from build123d import *

# Parameters (mm, degrees)
SKIZZE1_W                        = 150
SKIZZE1_H                        = 150
AUFSATZ_LINEAR_AUSTRAGEN1_DEPTH  = 2
AUFSATZ_LINEAR_AUSTRAGEN2_DEPTH  = 80
SCHNITT_LINEAR_AUSTRAGEN1_DEPTH  = 10
SKIZZE5_W                        = 17
SKIZZE5_H                        = 13
SCHNITT_LINEAR_AUSTRAGEN3_DEPTH  = 10
SKIZZE6_W                        = 17
SKIZZE6_H                        = 19
SCHNITT_LINEAR_AUSTRAGEN4_DEPTH  = 2
SKIZZE7_W                        = 17
SKIZZE7_H                        = 3
SCHNITT_LINEAR_AUSTRAGEN5_DEPTH  = 10
SKIZZE9_W                        = 18
SKIZZE9_H                        = 21
AUFSATZ_LINEAR_AUSTRAGEN3_DEPTH  = 63
SKIZZE10_W                       = 15
SKIZZE10_H                       = 10
SCHNITT_LINEAR_AUSTRAGEN6_DEPTH  = 63
SCHNITT_LINEAR_AUSTRAGEN7_DEPTH  = 2
SKIZZE17_R                       = 1
SCHNITT_LINEAR_AUSTRAGEN10_DEPTH = 1
SKIZZE18_W                       = 7
SKIZZE18_H                       = 7
SCHNITT_LINEAR_AUSTRAGEN11_DEPTH = 4.5
SKIZZE19_R                       = 0.9
SCHNITT_LINEAR_AUSTRAGEN12_DEPTH = 15
SKIZZE20_W                       = 25
SKIZZE20_H                       = 37
SCHNITT_LINEAR_AUSTRAGEN13_DEPTH = 4
SKIZZE21_W                       = 7
SKIZZE21_H                       = 37
SCHNITT_LINEAR_AUSTRAGEN14_DEPTH = 3
SCHNITT_LINEAR_AUSTRAGEN15_DEPTH = 6


with BuildPart() as part:
    # Skizze1 → Aufsatz-Linear austragen1 (new body)
    with BuildSketch(Plane(origin=(0, 0, 0), x_dir=(1, 0, 0), z_dir=(0, 1, 0))):
        with Locations((-0.733702775, 32.058376742)):
            Rectangle(SKIZZE1_W, SKIZZE1_H)
    extrude(amount=-AUFSATZ_LINEAR_AUSTRAGEN1_DEPTH)

    # Skizze1_3 → Aufsatz-Linear austragen2 (add)
    with BuildSketch(Plane(origin=(0, 0, 0), x_dir=(1, 0, 0), z_dir=(0, 1, 0))):
        Polygon((-75.733702775, 107.058376742), (-75.733702775, 48.496785112), (-70.733702775, 48.496785112), (-70.733702775, 105.058376742), (69.266297225, 105.058376742), (69.266297225, 56.802887669), (74.266297225, 56.802887669), (74.266297225, 107.058376742), align=None)
        Polygon((-15.65559864, -40.941623258), (-15.65559864, -42.941623258), (74.266297225, -42.941623258), (74.266297225, 56.802887669), (69.266297225, 56.802887669), (69.266297225, -40.941623258), align=None)
        Polygon((-70.733702775, 48.496785112), (-75.733702775, 48.496785112), (-75.733702775, -42.941623258), (-15.65559864, -42.941623258), (-15.65559864, -40.941623258), (-70.733702775, -40.941623258), align=None)
    extrude(amount=AUFSATZ_LINEAR_AUSTRAGEN2_DEPTH)

    # Skizze2 → Schnitt-Linear austragen1 (cut)
    with BuildSketch(Plane.ZY.offset(75.733702775)):
        Polygon((-75.558376742, 67.5), (-75.558376742, 62.78), (-32.058376742, 39), (11.441623258, 62.78), (11.441623258, 67.5), align=None)
        Polygon((-32.058376742, 39), (-75.558376742, 62.78), (-75.558376742, 15.22), align=None)
        Polygon((11.441623258, 15.22), (-32.058376742, 39), (-75.558376742, 15.22), (-75.558376742, 10.5), (11.441623258, 10.5), align=None)
        Polygon((11.441623258, 62.78), (-32.058376742, 39), (11.441623258, 15.22), align=None)
    extrude(amount=-SCHNITT_LINEAR_AUSTRAGEN1_DEPTH, mode=Mode.SUBTRACT)

    # Skizze5 → Schnitt-Linear austragen3 (cut)
    with BuildSketch(Plane(origin=(74.266297225, 0, 0), x_dir=(0, 0, -1), z_dir=(1, 0, 0))):
        with Locations((93.558376742, 68.5)):
            Rectangle(SKIZZE5_W, SKIZZE5_H)
    extrude(amount=-SCHNITT_LINEAR_AUSTRAGEN3_DEPTH, mode=Mode.SUBTRACT)

    # Skizze6 → Schnitt-Linear austragen4 (cut)
    with BuildSketch(Plane(origin=(74.266297225, 0, 0), x_dir=(0, 0, -1), z_dir=(1, 0, 0))):
        with Locations((-29.441623258, 65.5)):
            Rectangle(SKIZZE6_W, SKIZZE6_H)
    extrude(amount=-SCHNITT_LINEAR_AUSTRAGEN4_DEPTH, mode=Mode.SUBTRACT)

    # Skizze7 → Schnitt-Linear austragen5 (cut)
    with BuildSketch(Plane(origin=(72.266297225, 0, 0), x_dir=(0, 0, -1), z_dir=(1, 0, 0))):
        with Locations((-29.441623258, 73.5)):
            Rectangle(SKIZZE7_W, SKIZZE7_H)
    extrude(amount=-SCHNITT_LINEAR_AUSTRAGEN5_DEPTH, mode=Mode.SUBTRACT)

    # Skizze9 → Aufsatz-Linear austragen3 (add)
    with BuildSketch(Plane(origin=(0, 0, 0), x_dir=(1, 0, 0), z_dir=(0, 1, 0))):
        with Locations((60.266297225, 94.558376742)):
            Rectangle(SKIZZE9_W, SKIZZE9_H)
    extrude(amount=AUFSATZ_LINEAR_AUSTRAGEN3_DEPTH)

    # Skizze10 → Schnitt-Linear austragen6 (cut)
    with BuildSketch(Plane(origin=(0, 0, 40.941623258), x_dir=(-1, 0, 0), z_dir=(0, 0, -1))):
        with Locations((-61.766297225, 5)):
            Rectangle(SKIZZE10_W, SKIZZE10_H)
    extrude(amount=-SCHNITT_LINEAR_AUSTRAGEN6_DEPTH, mode=Mode.SUBTRACT)

    # Skizze11 → Schnitt-Linear austragen7 (cut)
    with BuildSketch(Plane(origin=(-70.733702775, 0, 0), x_dir=(0, 0, -1), z_dir=(1, 0, 0))):
        Polygon((75.558376742, 16.164383562), (32.058376742, 40), (-11.441623258, 16.164383562), (-11.441623258, 10.5), (75.558376742, 10.5), align=None)
        Polygon((75.558376742, 63.835616438), (32.058376742, 40), (75.558376742, 16.164383562), align=None)
        Polygon((-11.441623258, 67.5), (-11.441623258, 63.835616438), (32.058376742, 40), (75.558376742, 63.835616438), (75.558376742, 67.5), align=None)
        Polygon((32.058376742, 40), (-11.441623258, 63.835616438), (-11.441623258, 16.164383562), align=None)
        Polygon((-11.441623258, 63.835616438), (-18.441623258, 67.671232877), (-18.441623258, 12.328767123), (-11.441623258, 16.164383562), align=None)
        Polygon((-18.441623258, 72.5), (-18.441623258, 67.671232877), (-11.441623258, 63.835616438), (-11.441623258, 67.5), (75.558376742, 67.5), (75.558376742, 63.835616438), (82.558376742, 67.671232877), (82.558376742, 72.5), align=None)
        Polygon((75.558376742, 63.835616438), (75.558376742, 16.164383562), (82.558376742, 12.328767123), (82.558376742, 67.671232877), align=None)
        Polygon((-11.441623258, 16.164383562), (-18.441623258, 12.328767123), (-18.441623258, 7.5), (82.558376742, 7.5), (82.558376742, 12.328767123), (75.558376742, 16.164383562), (75.558376742, 10.5), (-11.441623258, 10.5), align=None)
    extrude(amount=-SCHNITT_LINEAR_AUSTRAGEN7_DEPTH, mode=Mode.SUBTRACT)

    # Skizze17 → Schnitt-Linear austragen10 (cut)
    with BuildSketch(Plane(origin=(-72.733702775, 0, 0), x_dir=(0, 0, -1), z_dir=(1, 0, 0))):
        with Locations((77.758376742, 67)):
            Circle(SKIZZE17_R)
        with Locations((77.758376742, 11)):
            Circle(SKIZZE17_R)
        with Locations((-13.641623258, 11)):
            Circle(SKIZZE17_R)
        with Locations((-13.641623258, 67)):
            Circle(SKIZZE17_R)
    extrude(amount=-SCHNITT_LINEAR_AUSTRAGEN10_DEPTH, mode=Mode.SUBTRACT)

    # Skizze18 → Schnitt-Linear austragen11 (cut)
    with BuildSketch(Plane.ZY.offset(75.733702775)):
        with Locations((27.191623258, 57.5)):
            Rectangle(SKIZZE18_W, SKIZZE18_H)
        Polygon((30.691623258, 31), (27.191623258, 31), (23.691623258, 31), (23.691623258, 24), (30.691623258, 24), align=None)
        with Locations((27.191623258, 37.5)):
            Rectangle(SKIZZE18_W, SKIZZE18_H)
        with Locations((27.191623258, 47.5)):
            Rectangle(SKIZZE18_W, SKIZZE18_H)
        with Locations((-91.518407477, 57.5)):
            Rectangle(SKIZZE18_W, SKIZZE18_H)
        with Locations((-91.518407477, 47.5)):
            Rectangle(SKIZZE18_W, SKIZZE18_H)
        with Locations((-91.518407477, 37.5)):
            Rectangle(SKIZZE18_W, SKIZZE18_H)
        with Locations((-91.518407477, 27.5)):
            Rectangle(SKIZZE18_W, SKIZZE18_H)
    extrude(amount=-SCHNITT_LINEAR_AUSTRAGEN11_DEPTH, mode=Mode.SUBTRACT)

    # Skizze19 → Schnitt-Linear austragen12 (cut)
    with BuildSketch(Plane(origin=(0, 80, 0), x_dir=(1, 0, 0), z_dir=(0, 1, 0))):
        with BuildLine():
            Line((72.666297225, 7.058376742), (71.766297225, 7.058376742))
            Line((71.766297225, 7.058376742), (71.766297225, 6.158376742))
            ThreePointArc((71.766297225, 6.158376742), (72.402693328, 6.421980639), (72.666297225, 7.058376742))
        make_face()
        with BuildLine():
            Line((71.766297225, 6.158376742), (71.766297225, 7.058376742))
            Line((71.766297225, 7.058376742), (70.866297225, 7.058376742))
            ThreePointArc((70.866297225, 7.058376742), (71.129901122, 6.421980639), (71.766297225, 6.158376742))
        make_face()
        with BuildLine():
            Line((70.866297225, 7.058376742), (71.766297225, 7.058376742))
            Line((71.766297225, 7.058376742), (72.666297225, 7.058376742))
            ThreePointArc((72.666297225, 7.058376742), (71.766297225, 7.958376742), (70.866297225, 7.058376742))
        make_face()
        with Locations(Location((71.766297225, 57.058376742, 0), (0, 0, 270))):
            Circle(SKIZZE19_R)
        with Locations(Location((-73.233702775, -32.941623258, 0), (0, 0, 270))):
            Circle(SKIZZE19_R)
        with Locations(Location((-73.233702775, 97.058376742, 0), (0, 0, 270))):
            Circle(SKIZZE19_R)
    extrude(amount=-SCHNITT_LINEAR_AUSTRAGEN12_DEPTH, mode=Mode.SUBTRACT)

    # Skizze20 → Schnitt-Linear austragen13 (cut)
    with BuildSketch(Plane(origin=(74.266297225, 0, 0), x_dir=(0, 0, -1), z_dir=(1, 0, 0))):
        with Locations((32.058376742, 56.476963809)):
            Rectangle(SKIZZE20_W, SKIZZE20_H)
    extrude(amount=-SCHNITT_LINEAR_AUSTRAGEN13_DEPTH, mode=Mode.SUBTRACT)

    # Skizze21 → Schnitt-Linear austragen14 (cut)
    with BuildSketch(Plane(origin=(70.266297225, 0, 0), x_dir=(0, 0, -1), z_dir=(1, 0, 0))):
        with Locations((23.058376742, 56.476963809)):
            Rectangle(SKIZZE21_W, SKIZZE21_H)
    extrude(amount=-SCHNITT_LINEAR_AUSTRAGEN14_DEPTH, mode=Mode.SUBTRACT)

    # Skizze24 → Schnitt-Linear austragen15 (cut)
    with BuildSketch(Plane(origin=(70.266297225, 0, 0), x_dir=(0, 0, -1), z_dir=(1, 0, 0))):
        with BuildLine():
            ThreePointArc((42.058376742, 39.976963809), (42.411930132, 40.123410418), (42.558376742, 40.476963809))
            Line((42.558376742, 40.476963809), (42.058376742, 40.476963809))
            Line((42.058376742, 40.476963809), (42.058376742, 39.976963809))
        make_face()
        with BuildLine():
            Line((42.058376742, 40.476963809), (42.558376742, 40.476963809))
            ThreePointArc((42.558376742, 40.476963809), (41.704823351, 40.830517199), (42.058376742, 39.976963809))
            Line((42.058376742, 39.976963809), (42.058376742, 40.476963809))
        make_face()
    extrude(amount=-SCHNITT_LINEAR_AUSTRAGEN15_DEPTH, mode=Mode.SUBTRACT)


solid = part.part
For this review, take the finished solid that the model builds, in its own axes (mm). A direction names the side the tool comes from. Round coordinates to 2 decimals unless told otherwise and drop trailing zeros. Order: outer loops, then holes, each group sorted by start corner. A loop starts at its lowest first (then second) coordinate and runs counter-clockwise, first axis right, second up. Notation, with made-up numbers: M -11,-22.75 L 10,-22.75 A11 ccw 10,-12.75 Z; hole C -17.5,-19 d3. An arc over 180 degrees is marked long. Use a Markdown table: item, result. Add a question column.
Item 1: Insertion check: pin 1 (5.5 mm diameter, centred on y = 39, z = -92, fed in from -X); pin 2 (1 mm diameter, centred on x = 37.5, z = -5.5, fed in from +Y); pin 3 (8 mm diameter, centred on y = 40.5, z = -51.5, fed in from -X); pin 4 (12 mm diameter, centred on x = 50.5, z = -88.5, fed in from +Y). Each pin has a flat end and moves straight along its axis. Give the tip position at first contact, or say it passes through.
Item 2: Add section B-B, the plane y = 3. Give the boundary of the cut face in (x, z), then the cut area to 3 significant figures.
Item 3: Add section C-C, the plane x = 13.5. Give the boundary of the cut face in (y, z).
Item 4: To check wall thickness, follow line 1 along X through (y, z) = (71.5, -77); line 2 along Z through (x, y) = (65.5, 52); line 3 along Z through (x, y) = (-57.5, 74). State the ranges of each line that lie inside material, in increasing order.
Item 5: Mouldability with a two-part tool opening along Z and no side actions: class faces 1 (the flat face through (-2, 38, 42.942)), 2 (the flat face through (60, 63, -95)) as released by +Z, released by -Z, zero draft, split by the parting line, or undercut.
Item 6: Tool access review of faces 3 (the flat face through (-74, 27, 30.692)), 4 (the flat face through (70.266, 57, -35)): name each direction out of +Z, -Z, +X, -X, +Y, -Y from which nothing blocks a thin tool from reaching the whole face with its end or side.
Item 7: Add section A-A, the plane z = -52. Give the boundary of the cut face in (x, y).
Geometry results:
| question | item | result |
|---|---|---|
| 1 | pin 1 | stops at x = -75.73 |
| 1 | pin 2 | stops at y = 0 |
| 1 | pin 3 | stops at x = 69.27 |
| 1 | pin 4 | stops at y = 63 |
| 2 | outline | M -75.73,-107.06 L 74.27,-107.06 L 74.27,42.94 L 69.27,42.94 L 69.27,-84.06 L 51.27,-84.06 L 51.27,-105.06 L -70.73,-105.06 L -70.73,40.94 L 54.27,40.94 L 54.27,42.94 L -75.73,42.94 Z |
| 2 | area | 2,410 mm² |
| 3 | outline | M -2,-107.06 L 80,-107.06 L 80,-105.06 L 0,-105.06 L 0,40.94 L 80,40.94 L 80,42.94 L -2,42.94 Z |
| 4 | line 1 | x = -75.73 to -72.73, 69.27 to 74.27 |
| 4 | line 2 | z = -107.06 to -84.06, 40.94 to 42.94 |
| 4 | line 3 | z = -107.06 to -105.06, 40.94 to 42.94 |
| 5 | face 1 | released by +Z |
| 5 | face 2 | undercut |
| 6 | face 3 | -X |
| 6 | face 4 | +X |
| 7 | outline | M -75.73,-2 L 74.27,-2 L 74.27,80 L 69.27,80 L 69.27,0 L -70.73,0 L -70.73,7.5 L -72.73,7.5 L -72.73,10.5 L -75.73,10.5 Z; M -75.73,67.5 L -72.73,67.5 L -72.73,72.5 L -70.73,72.5 L -70.73,80 L -75.73,80 Z |
